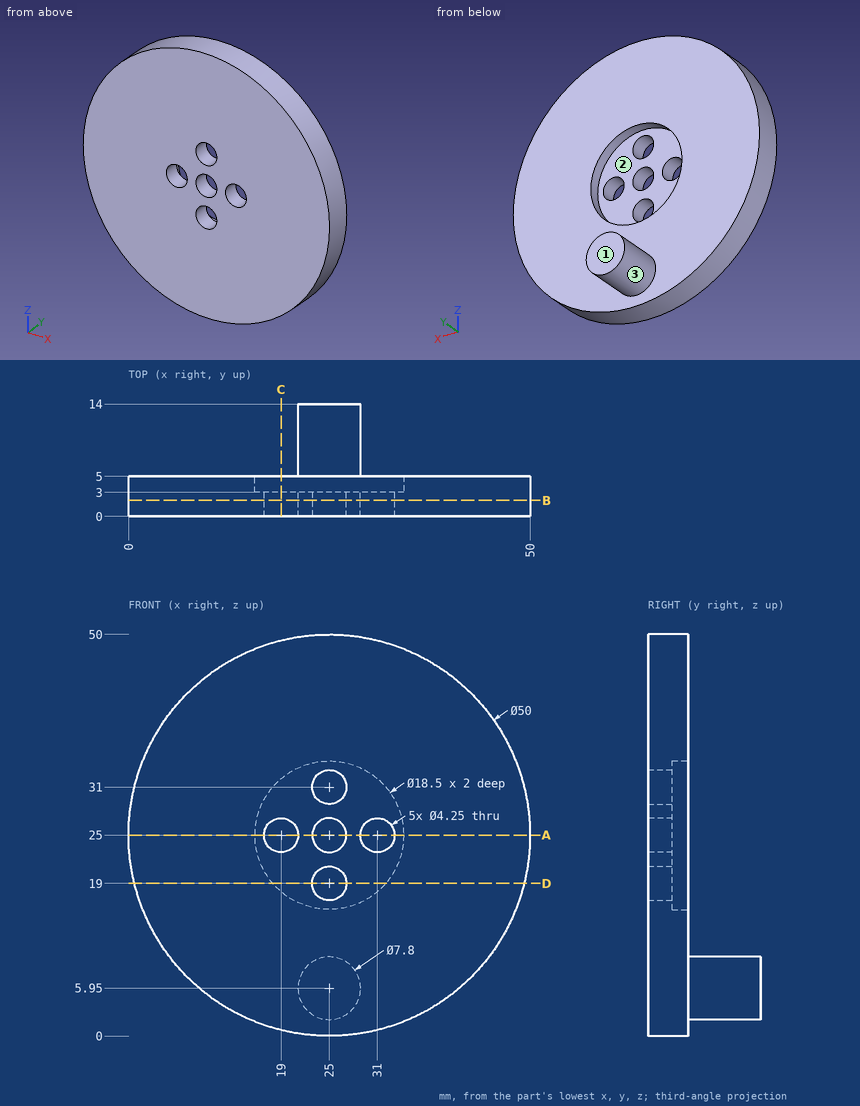
Study the drawing (mm; zero at the part's minimum x, y, z) and answer. Give positions to 0.01 mm unless a question says otherwise; leave off trailing zeros. Write each loop counter-clockwise with the first axis right and the second up, starting at its lowest first coordinate (ties: lowest second). Pieces come first, ordered by that corner, then holes. Notation, with made-up numbers: (60, 0) -> (71, 0) arc R25 ccw to (71, 39) -> close; hole circle Ø4 at (41.5, -26). An arc over 180 degrees is marked (long way). Answer in a Markdown table with one row per item.
1) Each of these flat-tipped pins is pushed along its axis until it touches: pin 1 Ø2 at (x, y) = (5, 2.5) entering from -Z; pin 2 Ø8 at (x, y) = (10, 4.5) entering from -Z; pin 3 Ø5.5 at (x, z) = (19, 25) entering from +Y; pin 4 Ø3.5 at (x, z) = (25, 25) entering from -Y. Where does it stop, or does it pass through?
Results list:
| item | result |
|---|---|
| pin 1 | z = 8.75 |
| pin 2 | z = 2.55 |
| pin 3 | y = 3 |
| pin 4 | through |
2) Section B-B on y = 2 is taken. Give the vertices of the cut face in (x, z) (3 decimals).
Results list:
| item | result |
|---|---|
| outline | circle Ø50 at (25, 25); hole circle Ø4.25 at (19, 25); hole circle Ø4.25 at (25, 19); hole circle Ø4.25 at (25, 25); hole circle Ø4.25 at (25, 31); hole circle Ø4.25 at (31, 25) |
3) Straight lines are drawn through the part: line 1 (Z direction, x = 25, y = 1.4) (3 decimals); line 2 (Y direction, x = 40.5, z = 12); line 3 (X direction, y = 1.85, z = 31) (3 decimals). For each, find the intervals that lie inside material, in ascending order. Write a range as [from, to].
Results list:
| item | result |
|---|---|
| line 1 | [0, 16.875], [21.125, 22.875], [27.125, 28.875], [33.125, 50] |
| line 2 | [0, 5] |
| line 3 | [0.731, 22.875], [27.125, 49.269] |
4) Section C-C on x = 19 is taken. Give the vertices of the cut face in (y, z) (3 decimals), plus the area to 3 significant figures.
Results list:
| item | result |
|---|---|
| outline | (0, 0.731) -> (5, 0.731) -> (5, 17.96) -> (3, 17.96) -> (3, 22.875) -> (0, 22.875) -> close; (0, 27.125) -> (3, 27.125) -> (3, 32.04) -> (5, 32.04) -> (5, 49.269) -> (0, 49.269) -> close |
| area | 202 mm^2 |
5) Section A-A on z = 25 is taken. Give the vertices of the cut face in (x, y) (3 decimals).
Results list:
| item | result |
|---|---|
| outline | (0, 0) -> (16.875, 0) -> (16.875, 3) -> (15.75, 3) -> (15.75, 5) -> (0, 5) -> close; (21.125, 0) -> (22.875, 0) -> (22.875, 3) -> (21.125, 3) -> close; (27.125, 0) -> (28.875, 0) -> (28.875, 3) -> (27.125, 3) -> close; (33.125, 0) -> (50, 0) -> (50, 5) -> (34.25, 5) -> (34.25, 3) -> (33.125, 3) -> close |
6) Determine the mould class of the marked faces 1, 2 and 3 for opening direction Z: released by +Z, released by -Z, zero draft, split by the parting line, or undercut.
Results list:
| item | result |
|---|---|
| face 1 | zero draft |
| face 2 | undercut |
| face 3 | split by the parting line |
7) Section D-D on z = 19 is taken. Give the vertices of the cut face in (x, y) (3 decimals).
Results list:
| item | result |
|---|---|
| outline | (0.731, 0) -> (22.875, 0) -> (22.875, 3) -> (17.96, 3) -> (17.96, 5) -> (0.731, 5) -> close; (27.125, 0) -> (49.269, 0) -> (49.269, 5) -> (32.04, 5) -> (32.04, 3) -> (27.125, 3) -> close |
